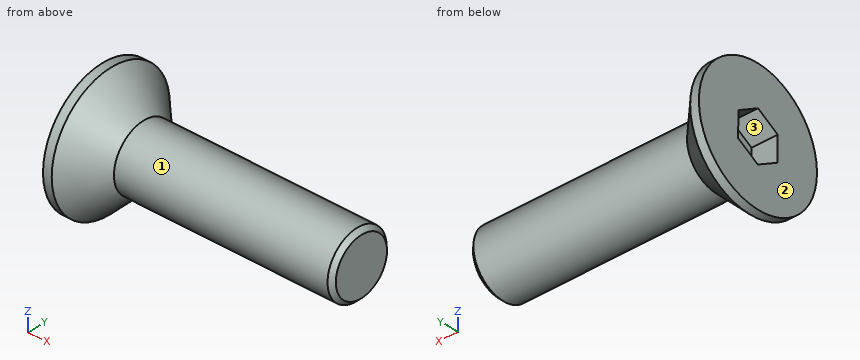
Autodesk Inventor part; units mm, degrees
ref_plane "YZ Plane" through (0, 0, 0) normal (1, 0, 0) x (0, 1, 0)
ref_plane "XZ Plane" through (0, 0, 0) normal (0, 1, 0) x (-1, 0, 0)
ref_plane "XY Plane" through (0, 0, 0) normal (0, 0, 1) x (1, 0, 0)
sketch "Sketch1" plane through (0, 0, 0) normal (0, 0, 1) x (1, 0, 0)
  line L0 (0, 0) -> (0, 3)
  line L1 (0, 3) -> (0.4, 3)
  line L2 (0.4, 3) -> (1.9, 1.5)
  line L3 (1.9, 1.5) -> (11.9, 1.5)
  line L4 (11.9, 1.5) -> (11.9, 0)
  line L5 (11.9, 0) -> (0, 0)
  dimension "d0" = 10
  dimension "d1" = 45
  dimension "d2" = 1.9
  dimension "d3" = 1.5
  dimension "d4" = 3
revolve "Revolution1" add sketch "Sketch1" angle 360 about axis through (11.9, 0, 0) along (-1, 0, 0)
sketch "Sketch2" plane through (0, 0, 0) normal (-1, 0, 0) x (0, 0, 1)
  line L0 (0.5725, -1.0028) -> (-0.5822, -0.9972)
  line L1 (-0.5822, -0.9972) -> (-1.1547, 0.0056)
  line L2 (-1.1547, 0.0056) -> (-0.5725, 1.0028)
  line L3 (-0.5725, 1.0028) -> (0.5822, 0.9972)
  line L4 (0.5822, 0.9972) -> (1.1547, -0.0056)
  line L5 (1.1547, -0.0056) -> (0.5725, -1.0028)
  point P0 (0, 0)
  point P1 (0, 0)
  dimension "d6" = 2
extrude "Extrusion1" cut sketch "Sketch2" against normal blind 1.2
thread "Thread1"
chamfer "Chamfer1" distance 0.2 angle 45 1 edges at (11.9, -1.5, 0)
properties part number "M3 x 10 mm FHCS"
CAD build for the part. Positions are in the model's coordinates, mm. Face numbers are marked on the shaded views. Round coordinates to 2 decimals unless told otherwise and drop trailing zeros. Write each loop counter-clockwise with the first axis right and the second up, starting at its lowest first coordinate (ties: lowest second). Pieces come first, ordered by that corner, then holes. Notation, with made-up numbers: (4, 19) -> (30, 19) arc R5 cw to (30, 26) -> close; hole circle Ø3 at (64.25, -11). An arc over 180 degrees is marked (long way). Answer in a Markdown table with one row per item. Add a question column.
Item 1: Saw through at B-B, the plane x = 11. Write the cut outline in (y, z).
Item 2: Saw through at A-A, the plane z = 0. Write the cut outline in (x, y), then the cut area to 3 significant figures.
Item 3: Drill centre lines: line 1 (X direction, y = -0.05, z = -0.65); line 2 (X direction, y = 0.45, z = 2.2); line 3 (Z direction, x = 2.5, y = -0.1). Where is each one in solid material? Low to high. Write a range as from..to.
Item 4: Drop flat-ended pins along their axis: pin 1 Ø1 at (y, z) = (0, 0.5) entering from -X; pin 2 Ø1.5 at (x, z) = (2, 1) entering from +Y. Give the stop position or say it passes through.
Item 5: Mould opens along Z. For the marked faces 1, 2 and 3 say: pulls with the +Z half, pulls with the -Z half, needs draft (parallel to the pull), parting line crosses it, or undercut.
Findings below:
| question | item | result |
|---|---|---|
| 1 | outline | circle Ø3 at (0, 0) |
| 2 | outline | (0, -3) -> (0.4, -3) -> (1.9, -1.5) -> (11.7, -1.5) -> (11.9, -1.3) -> (11.9, 1.3) -> (11.7, 1.5) -> (1.9, 1.5) -> (0.4, 3) -> (0, 3) -> (0, 1) -> (1.2, 1) -> (1.2, -1) -> (0, -1) -> close |
| 2 | area | 36.7 mm^2 |
| 3 | line 1 | x = 1.2..11.9 |
| 3 | line 2 | x = 0..1.15 |
| 3 | line 3 | z = -1.5..1.5 |
| 4 | pin 1 | stops at x = 1.2 |
| 4 | pin 2 | stops at y = 1.97 |
| 5 | face 1 | parting line crosses it |
| 5 | face 2 | needs draft |
| 5 | face 3 | undercut |
